Check sheet for the modelled part. Datum: model origin and axes. Units: mm. Give positions to 0.01 mm unless a question says otherwise; leave off trailing zeros. Order: outer loops, then holes, each group sorted by start corner. A loop starts at its lowest first (then second) coordinate and runs counter-clockwise, first axis right, second up. Notation, with made-up numbers: M 4,13.5 L 37,13.5 A20 cw 37,28.5 Z; hole C 8,7 d4. An arc over 180 degrees is marked long. One line per question, with ' | ' between items. Start each with the question number.
Autodesk Inventor part; units mm, degrees
ref_plane "YZ Plane" through (0, 0, 0) normal (1, 0, 0) x (0, 1, 0)
ref_plane "XZ Plane" through (0, 0, 0) normal (0, 1, 0) x (-1, 0, 0)
ref_plane "XY Plane" through (0, 0, 0) normal (0, 0, 1) x (1, 0, 0)
sketch "Sketch1" plane through (0, 0, 0) normal (0, 0, 1) x (1, 0, 0)
  line L0 (-15, 7.5) -> (15, 7.5)
  line L1 (15, 7.5) -> (15, -7.5)
  line L2 (15, -7.5) -> (-15, -7.5)
  line L3 (-15, -7.5) -> (-15, 7.5)
  line L4 (-15, 7.5) -> (15, -7.5) construction
  line L5 (15, 7.5) -> (-15, -7.5) construction
  circle A0 centre (-12, 4.5) radius 2
  line L6 (0, -7.5) -> (0, 7.5)
  circle A1 centre (12, 4.5) radius 2
  point P0 (0, 0)
  dimension "d0" = 4
  dimension "d1" = 3
  dimension "d2" = 3
  dimension "d3" = 30
  dimension "d4" = 15
  dimension "d5" = 24
extrude "Extrusion1" add sketch "Sketch1" along normal blind 3
properties part number "imu_holder"
Item 1: Section check C-C, the plane z = 0.4. Record the cut outline in (x, y).
Item 2: Section check A-A, the plane x = 12. Record the cut outline in (y, z), then the cut area to 3 significant figures.
Item 3: Section check B-B, the plane y = 4.5. Record the cut outline in (x, z).
Item 4: Go/stop test with a flat-tipped pin: P1, Ø2.5, axis at x = -12, y = 4.5, coming from the +Z side. Record where the tip stops, or that it passes through.
Item 5: Scan lines: probe 1 along Y at (x, z) = (-12, 1.75); probe 2 along Y at (x, z) = (-13, 0.8); probe 3 along X at (y, z) = (4.75, 0.2). Record each from-to range of solid material in increasing order. Write a range as [from, to].
Item 6: Draft check along X on faces 1 (the face through (-13.6, 5.7, 1.5)), 2 (the face through (0, 0, 3)), 3 (the face through (-15, 0, 1)). Enter one of: released by +X, released by -X, zero draft, split by the parting line, or undercut.
Reported:
1) outline: M -15,-7.5 L 15,-7.5 L 15,7.5 L -15,7.5 Z; hole C -12,4.5 d4; hole C 12,4.5 d4
2) outline: M -7.5,0 L 2.5,0 L 2.5,3 L -7.5,3 Z; M 6.5,0 L 7.5,0 L 7.5,3 L 6.5,3 Z | area: 33.0 mm^2
3) outline: M -15,0 L -14,0 L -14,3 L -15,3 Z; M -10,0 L 10,0 L 10,3 L -10,3 Z; M 14,0 L 15,0 L 15,3 L 14,3 Z
4) P1: passes through
5) probe 1: y = [-7.5, 2.5], [6.5, 7.5] | probe 2: y = [-7.5, 2.77], [6.23, 7.5] | probe 3: x = [-15, -13.98], [-10.02, 10.02], [13.98, 15]
6) face 1: undercut | face 2: zero draft | face 3: released by -X
